Build history of the part. All positions in model axes, mm. A direction names the side the tool comes from. Round coordinates to 2 decimals unless told otherwise and drop trailing zeros. Loops run counter-clockwise (first coordinate to the right, second up) from the corner with the lowest first, then second, coordinate; pieces in that order, holes last. Notation, with made-up numbers: M 52,62 L 84,62 A21 cw 84,79 Z; hole C -39.75,-21.75 d9. An arc over 180 degrees is marked long. One line per item, written item: value.
```python
from build123d import *

# Parameters (mm, degrees)
SKETCH_2_R               = 2.75
CUT_EXTRUDE_1_DEPTH      = 37.742346142
CUT_EXTRUDE_START        = 20
CUT_EXTRUDE_2_DEPTH      = 20
PATTERN_CIRCULAR_1_COUNT = 16
CHAMFER_1_SIZE           = 0.3


with BuildPart() as part:
    # Эскиз1 → Повернуть1 (revolve)
    with BuildSketch(Plane.XY, mode=Mode.PRIVATE) as revolve_1_sk:
        Polygon((0, 6), (0, 15), (-5, 15), (-5, 12.5), (-25, 12.5), (-25, 15), (-30, 15), (-30, 6), align=None)
    revolve(revolve_1_sk.sketch.rotate(Axis((-33.310992453, 0, 0), (1, 0, 0)), 90), axis=Axis((-33.310992453, 0, 0), (1, 0, 0)))

    # Эскиз2 → Вырез-Вытянуть1 (cut, through all)
    with BuildSketch(Plane(origin=(0, 0, 0), x_dir=(1, 0, 0), z_dir=(0, 1, 0))):
        with Locations(Location((-12, 0, 0), (0, 0, 270))):
            Circle(SKETCH_2_R)
    extrude(amount=-CUT_EXTRUDE_1_DEPTH, mode=Mode.SUBTRACT)

    # Эскиз3 → Вырез-Вытянуть2 (cut)
    with BuildSketch(Plane.ZY.offset(5).offset(CUT_EXTRUDE_START)):
        with BuildLine():
            Line((-1.5, 12.409673646), (-1, 11))
            Line((-1, 11), (1, 11))
            Line((1, 11), (1.5, 12.409673646))
            ThreePointArc((1.5, 12.409673646), (0, 12.5), (-1.5, 12.409673646))
        make_face()
    cut_extrude_2 = extrude(amount=-CUT_EXTRUDE_2_DEPTH, mode=Mode.SUBTRACT)

    # Круговой массив1: Вырез-Вытянуть2 ×16 about axis
    pattern_circular_1_axis = Axis((0, 0, 0), (1, 0, 0))
    for i in range(1, PATTERN_CIRCULAR_1_COUNT):
        add(cut_extrude_2.rotate(pattern_circular_1_axis, i * 360 / PATTERN_CIRCULAR_1_COUNT), mode=Mode.SUBTRACT)

    # Фаска1
    chamfer_1_edges = [part.edges().sort_by_distance(p)[0] for p in [
        (0, 0, -6),
        (-30, 0, -6),
        (-30, 0, -15),
        (-25, 0, -15),
        (-5, 0, -15),
        (0, 0, -15),
    ]]
    chamfer(chamfer_1_edges, length=CHAMFER_1_SIZE)


solid = part.part
```
Item 1: Wall check: line 1 along X through (y, z) = (-9.75, 0); line 2 along X through (y, z) = (9, -10.5); line 3 along Y through (x, z) = (-14.5, 10.5). Give the ranges that are in metal, low to high.
Check values:
line 1: x = -30 to -14.75, -9.25 to 0
line 2: x = -30 to -25, -5 to 0
line 3: y = -6.78 to -5.78, -3.4 to 3.4, 5.78 to 6.78
Item 2: Slice it at A-A, the plane z = 0. Give the number of separate pieces and of enclosed holes in the cut face, and give its area (3 significant figures).
Check values:
separate pieces: 3
enclosed holes: 0
area: 352 mm2
Item 3: Slice it at B-B, the plane y = 0. Give the cut face in (x, z), and give its area (3 significant figures).
Check values:
outline: M -30,-14.7 L -29.7,-15 L -25.3,-15 L -25,-14.7 L -25,-11 L -5,-11 L -5,-14.7 L -4.7,-15 L -0.3,-15 L 0,-14.7 L 0,-6.3 L -0.3,-6 L -29.7,-6 L -30,-6.3 Z; M -30,6.3 L -29.7,6 L -0.3,6 L 0,6.3 L 0,14.7 L -0.3,15 L -4.7,15 L -5,14.7 L -5,11 L -25,11 L -25,14.7 L -25.3,15 L -29.7,15 L -30,14.7 Z
area: 379 mm2
Item 4: Pull direction Y, two halves, no side cores. Call faces 1 (the face through (-15.14, -12.257, 2.452)), 2 (the face through (-15.14, 3.324, 11.282)), 3 (the face through (-15.14, 2.43, -12.26)): pulls with the +Y half, pulls with the -Y half, needs draft (parallel to the pull), parting line crosses it, or undercut.
Check values:
face 1: pulls with the -Y half
face 2: undercut
face 3: pulls with the +Y half
Item 5: Which spindle directions (+Z, -Z, +X, -X, +Y, -Y) get a long thin tool onto all of the face, cutting with end or side? Do faces 4 (the face through (-7.38, -11.71, 1.25)), 5 (the face through (-15.14, 10.386, -6.956)), 6 (the face through (-15.14, -1.25, -11.71)), 7 (the face through (-15.1, 10.3, -5.6)), 8 (the face through (-5, -9, 8)). Say none if no direction does.
Check values:
face 4: -Y
face 5: -Z, +Y
face 6: -Z
face 7: +Y
face 8: none
Item 6: Drop flat-ended pins along their axis: P1, Ø1.6, axis at x = -17, y = 0, coming from the +Z side; P2, Ø1.5, axis at x = -8.5, z = 8.5, coming from the +Y side; P3, Ø10, axis at x = -5, y = 5.5, coming from the +Z side. Give the stop position or say it passes through.
Check values:
P1: stops at z = 11
P2: stops at y = 7.81
P3: stops at z = 14.99
Item 7: Slice it at C-C, the plane x = -26.5. Give the cut face in (y, z), and give its area (3 significant figures).
Check values:
outline: C 0,0 d30; hole C 0,0 d12
area: 594 mm2
